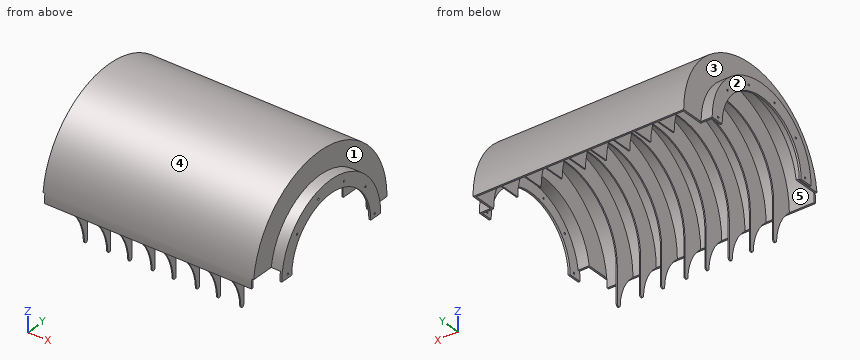
Autodesk Inventor part; units mm, degrees
ref_plane "YZ Plane" through (0, 0, 0) normal (1, 0, 0) x (0, 1, 0)
ref_plane "XZ Plane" through (0, 0, 0) normal (0, 1, 0) x (-1, 0, 0)
ref_plane "XY Plane" through (0, 0, 0) normal (0, 0, 1) x (1, 0, 0)
sketch "草图1" plane through (0, 0, 0) normal (0, 0, 1) x (1, 0, 0)
  circle A0 centre (0, 0) radius 141.3842
  line L0 (50, 166.3842) -> (50, 141.3842)
  line L1 (50, 141.3842) -> (-50, 141.3842)
  line L2 (-50, 141.3842) -> (-50, 166.3842)
  line L3 (-57.3473, 163.9969) -> (-42.6527, 143.7715)
  line L4 (-42.6527, 143.7715) -> (-123.5544, 84.9929)
  line L5 (-123.5544, 84.9929) -> (-138.249, 105.2184)
  line L6 (-142.7899, 98.9684) -> (-119.0135, 91.2429)
  line L7 (-119.0135, 91.2429) -> (-149.9152, -3.8627)
  line L8 (-149.9152, -3.8627) -> (-173.6916, 3.8627)
  line L9 (-173.6916, -3.8627) -> (-149.9152, 3.8627)
  line L10 (-149.9152, 3.8627) -> (-119.0135, -91.2429)
  line L11 (-119.0135, -91.2429) -> (-142.7899, -98.9684)
  line L12 (-138.249, -105.2184) -> (-123.5544, -84.9929)
  line L13 (-123.5544, -84.9929) -> (-42.6527, -143.7715)
  line L14 (-42.6527, -143.7715) -> (-57.3473, -163.9969)
  line L15 (-50, -166.3842) -> (-50, -141.3842)
  line L16 (-50, -141.3842) -> (50, -141.3842)
  line L17 (50, -141.3842) -> (50, -166.3842)
  line L18 (57.3473, -163.9969) -> (42.6527, -143.7715)
  line L19 (42.6527, -143.7715) -> (123.5544, -84.9929)
  line L20 (123.5544, -84.9929) -> (138.249, -105.2184)
  line L21 (142.7899, -98.9684) -> (119.0135, -91.2429)
  line L22 (119.0135, -91.2429) -> (149.9152, 3.8627)
  line L23 (149.9152, 3.8627) -> (173.6916, -3.8627)
  line L24 (173.6916, 3.8627) -> (149.9152, -3.8627)
  line L25 (149.9152, -3.8627) -> (119.0135, 91.2429)
  line L26 (119.0135, 91.2429) -> (142.7899, 98.9684)
  line L27 (138.249, 105.2184) -> (123.5544, 84.9929)
  line L28 (123.5544, 84.9929) -> (42.6527, 143.7715)
  line L29 (42.6527, 143.7715) -> (57.3473, 163.9969)
  line L30 (11.529, 166.3842) -> (50, 166.3842)
  line L31 (-315, 173.8842) -> (-280, 173.8842)
  line L32 (-280, 173.8842) -> (-280, 168.8842)
  line L33 (-280, 168.8842) -> (-315, 168.8842)
  line L34 (-315, 168.8842) -> (-315, 173.8842)
  line L35 (-315, 168.8842) -> (-310, 168.8842)
  line L36 (-310, 168.8842) -> (-310, 138.8842)
  line L37 (-310, 138.8842) -> (-315, 138.8842)
  line L38 (-315, 138.8842) -> (-315, 168.8842)
  line L39 (-280, 173.8842) -> (-285, 173.8842)
  line L40 (-285, 173.8842) -> (-285, 235)
  line L41 (-285, 235) -> (-280, 235)
  line L42 (-280, 235) -> (-280, 173.8842)
  line L43 (-280, 235) -> (280, 235)
  line L44 (280, 235) -> (280, 230)
  line L45 (280, 230) -> (-280, 230)
  line L46 (-280, 230) -> (-280, 235)
  line L47 (280, 235) -> (285, 235)
  line L48 (285, 235) -> (285, 173.8842)
  line L49 (285, 173.8842) -> (280, 173.8842)
  line L50 (280, 173.8842) -> (280, 235)
  line L51 (280, 173.8842) -> (315, 173.8842)
  line L52 (315, 173.8842) -> (315, 168.8842)
  line L53 (315, 168.8842) -> (280, 168.8842)
  line L54 (280, 168.8842) -> (280, 173.8842)
  line L55 (315, 168.8842) -> (310, 168.8842)
  line L56 (310, 168.8842) -> (310, 138.8842)
  line L57 (310, 138.8842) -> (315, 138.8842)
  line L58 (315, 138.8842) -> (315, 168.8842)
  line L59 (-213, 230) -> (-210, 230)
  line L60 (-210, 230) -> (-210, 175)
  line L61 (-210, 175) -> (-213, 175)
  line L62 (-213, 175) -> (-213, 230)
  line L63 (-150, 230) -> (-147, 230)
  line L64 (-147, 230) -> (-147, 175)
  line L65 (-147, 175) -> (-150, 175)
  line L66 (-150, 175) -> (-150, 230)
  line L67 (-93, 230) -> (-90, 230)
  line L68 (-90, 230) -> (-90, 175)
  line L69 (-90, 175) -> (-93, 175)
  line L70 (-93, 175) -> (-93, 230)
  line L71 (-30, 230) -> (-27, 230)
  line L72 (-27, 230) -> (-27, 175)
  line L73 (-27, 175) -> (-30, 175)
  line L74 (-30, 175) -> (-30, 230)
  line L75 (27, 230) -> (30, 230)
  line L76 (30, 230) -> (30, 175)
  line L77 (30, 175) -> (27, 175)
  line L78 (27, 175) -> (27, 230)
  line L79 (90, 230) -> (93, 230)
  line L80 (93, 230) -> (93, 175)
  line L81 (93, 175) -> (90, 175)
  line L82 (90, 175) -> (90, 230)
  line L83 (147, 230) -> (150, 230)
  line L84 (150, 230) -> (150, 175)
  line L85 (150, 175) -> (147, 175)
  line L86 (147, 175) -> (147, 230)
  line L87 (210, 230) -> (213, 230)
  line L88 (213, 230) -> (213, 175)
  line L89 (213, 175) -> (210, 175)
  line L90 (210, 175) -> (210, 230)
  line L91 (-441, 0) -> (441, 0)
  point P0 (0, 141.3842)
  point P1 (-83.1035, 114.3822)
  point P2 (-134.4643, 43.6901)
  point P3 (-134.4643, -43.6901)
  point P4 (-83.1035, -114.3822)
  point P5 (0, -141.3842)
  point P6 (83.1035, -114.3822)
  point P7 (134.4643, -43.6901)
  point P8 (134.4643, 43.6901)
  point P9 (83.1035, 114.3822)
  point P10 (50, 153.8842)
  dimension "d0" = 100
  dimension "d1" = 25
  dimension "d4" = 360
  dimension "d6" = 35
  dimension "d7" = 2.5
  dimension "d8" = 5
  dimension "d9" = 280
  dimension "d10" = 5
  dimension "d11" = 30
  dimension "d12" = 5
  dimension "d13" = 235
  dimension "d14" = 560
  dimension "d15" = 5
  dimension "d16" = 5
  dimension "d17" = 35
  dimension "d18" = 5
  dimension "d19" = 5
  dimension "d20" = 3
  dimension "d21" = 210
  dimension "d22" = 3
  dimension "d23" = 60
  dimension "d24" = 55
  dimension "d25" = 3
  dimension "d26" = 3
  dimension "d27" = 3
  dimension "d28" = 3
  dimension "d29" = 3
  dimension "d30" = 3
  dimension "d31" = 120
  dimension "d32" = 60
  dimension "d33" = 120
  dimension "d34" = 60
  dimension "d35" = 120
  dimension "d36" = 60
revolve "旋转1" add sketch "草图1" angle 180 about axis through (-10, 0, 0) along (1, 0, 0) contours L31 L32 L33 L34 | L40 L41 L42 L31 | L33 L36 L37 L38 | L42 L43 L44 L45 | L45 L60 L61 L62 | L47 L48 L49 L50 L44 | L45 L64 L65 L66 | L88 L89 L90 L45 | L49 L51 L52 L53 L54 | L45 L68 L69 L70 | L84 L85 L86 L45 | L53 L58 L57 L56 | L45 L72 L73 L74 | L80 L81 L82 L45 | L45 L76 L77 L78
sketch "草图2" plane through (-315, 138.8842, 0) normal (-1, 0, 0) x (0, 0, 1)
  circle A0 centre (10, 13.7887) radius 2.5
  arc A1 (27.2318, 11.6729) -> (10, 13.7887) centre (0, -138.8842) ccw
  arc A2 (0, -277.7684) -> (0, 0) centre (0, -138.8842) ccw
  line L0 (0, 35) -> (0, 0)
  line L1 (10, 13.7887) -> (0, -138.8842)
  point P0 (0, -138.8842)
  dimension "d38" = 5
  dimension "d39" = 153
  dimension "d40" = 10
extrude "拉伸1" cut sketch "草图2" against normal through all
pattern_circular "环形阵列1" count 6 over 172.5 about axis through (-312.5, 0, 0) along (1, 0, 0) of "拉伸1"
sketch "草图3" plane through (285, -235, 0) normal (0, 0, -1) x (-1, 0, 0)
  line L0 (72, 60) -> (75, 60)
  line L1 (75, 60) -> (75, 5)
  line L2 (75, 5) -> (72, 5)
  line L3 (72, 5) -> (72, 60)
  line L4 (135, 60) -> (138, 60)
  line L5 (138, 60) -> (138, 5)
  line L6 (138, 5) -> (135, 5)
  line L7 (135, 5) -> (135, 60)
  line L8 (192, 60) -> (195, 60)
  line L9 (195, 60) -> (195, 5)
  line L10 (195, 5) -> (192, 5)
  line L11 (192, 5) -> (192, 60)
  line L12 (255, 60) -> (258, 60)
  line L13 (258, 60) -> (258, 5)
  line L14 (258, 5) -> (255, 5)
  line L15 (255, 5) -> (255, 60)
  line L16 (312, 60) -> (315, 60)
  line L17 (315, 60) -> (315, 5)
  line L18 (315, 5) -> (312, 5)
  line L19 (312, 5) -> (312, 60)
  line L20 (375, 60) -> (378, 60)
  line L21 (378, 60) -> (378, 5)
  line L22 (378, 5) -> (375, 5)
  line L23 (375, 5) -> (375, 60)
  line L24 (432, 60) -> (435, 60)
  line L25 (435, 60) -> (435, 5)
  line L26 (435, 5) -> (432, 5)
  line L27 (432, 5) -> (432, 60)
  line L28 (495, 60) -> (498, 60)
  line L29 (498, 60) -> (498, 5)
  line L30 (498, 5) -> (495, 5)
  line L31 (495, 5) -> (495, 60)
  line L32 (565, 5) -> (498, 5)
  line L33 (498, 5) -> (498, 60)
  line L34 (135, 60) -> (135, 5)
  point P0 (285, 235)
extrude "拉伸2" add sketch "草图3" along normal blind 100
sketch "草图4" plane through (213, 175, 0) normal (1, 0, 0) x (0, 0, -1)
  line L0 (100, -405) -> (100, -350)
  arc A0 (100, -360) -> (0, -405) centre (100, -493.6111) ccw
  line L1 (0, -405) -> (100, -405)
  line L2 (0, -410) -> (0, -348.8842)
  line L3 (100, -360) -> (100, -405)
  point P0 (0, -175)
  dimension "d48" = 10
extrude "拉伸3" cut sketch "草图4" against normal up to surface (426 mm away)
sketch "草图5" plane through (213, 175, 0) normal (1, 0, 0) x (0, 0, -1)
  circle A0 centre (94.9541, -355.0459) radius 5.0459
  line L0 (0, -350) -> (100, -350)
  line L1 (100, -350) -> (100, -360)
  arc A1 (100, -360) -> (0, -405) centre (100, -493.6111) ccw
  line L2 (94.9541, -350) -> (100, -350)
  line L3 (100, -350.2573) -> (100, -360)
  arc A2 (100, -360) -> (95.1377, -360.0885) centre (100, -493.6111) ccw
  point P0 (0, -175)
extrude "拉伸4" cut sketch "草图5" against normal up to surface (426 mm away) contours L1 A1 A0 | A0 L0 L1
sketch "草图6" plane through (285, -235, 0) normal (0, 0, -1) x (-1, 0, 0)
  line L0 (595, 0) -> (565, 0)
  line L1 (565, 0) -> (565, 96.1158)
  line L2 (565, 96.1158) -> (595, 96.1158)
  line L3 (595, 96.1158) -> (595, 0)
  line L4 (595, 96.1158) -> (595, 66.1158)
  line L5 (565, 66.1158) -> (565, 5)
  line L6 (0, 0) -> (570, 0)
  line L7 (600, 96.1158) -> (595, 96.1158)
  line L8 (-25, 96.1158) -> (5, 96.1158)
  line L9 (5, 96.1158) -> (5, 0)
  line L10 (5, 0) -> (-25, 0)
  line L11 (-25, 0) -> (-25, 96.1158)
  line L12 (-25, 66.1158) -> (-25, 96.1158)
  line L13 (-25, 96.1158) -> (-30, 96.1158)
  line L14 (5, 5) -> (5, 66.1158)
  point P0 (285, 235)
extrude "拉伸5" cut sketch "草图6" against normal blind 25
properties part number "主动轮护盖"
Verification items for the finished model (mm, model axes). Face numbers are marked on the shaded views. A direction names the side the tool comes from. Give positions to 0.01 mm unless a question says otherwise; leave off trailing zeros. Loops run counter-clockwise (first coordinate to the right, second up) from the corner with the lowest first, then second, coordinate; pieces in that order, holes last.
1. Go/stop test with flat-tipped pins: P1, Ø3, axis at x = 97.5, z = 53.5, coming from the +Y side; P2, Ø1.5, axis at x = -28, z = -67.5, coming from the +Y side; P3, Ø2, axis at x = -175.5, y = 105, coming from the -Z side; P4, Ø6.5, axis at y = -45.36, z = 146.12, coming from the -X side. Record where each tip stops, or that it passes through.
Derived:
P1: stops at y = 229.17
P2: stops at y = -175
P3: stops at z = 204.12
P4: stops at x = -315
2. Cross-section at B-B on x = 43.5. Record the cut outline in (y, z), and give its area (3 significant figures).
Derived:
outline: (-235, 0) - (-230, 0) arc R230 cw to (230, 0) - (235, 0) arc R235 ccw to start
area: 3,650 mm2
3. Tool access check on the marked faces 1 and 2. Record the directions out of +Z, -Z, +X, -X, +Y, -Y that give a thin tool (end or side, any length) a straight path to the whole face; none if there is none.
Derived:
face 1: +Z, +X
face 2: +Z, -Z, -X, +Y, -Y
4. Material ranges on probe 1 along Y at (x, z) = (-24.5, 75); probe 2 along Y at (x, z) = (129.5, 157.5); probe 3 along Z at (x, y) = (-108, 5), recorded low to high.
Derived:
probe 1: y = -222.71 to -217.43, 217.43 to 222.71
probe 2: y = -174.41 to -167.61, 167.61 to 174.41
probe 3: z = 229.95 to 234.95
5. Release check for a two-part mould opening along Y. For the marked faces 3, 4 and 5 record: +Y half, -Y half, draft (parallel to the pull), parting line (faces both ways), or undercut.
Derived:
face 3: draft
face 4: parting line
face 5: undercut
6. Cross-section at A-A on z = -21. Count the separate pieces of the cut face and the enclosed holes in it, and give its area (3 significant figures).
Derived:
separate pieces: 8
enclosed holes: 0
area: 861 mm2
